Geometry: final body of the model. Coordinates: model frame, mm. A direction names the side the tool comes from. Round coordinates to 2 decimals unless told otherwise and drop trailing zeros. Loops run counter-clockwise (first coordinate to the right, second up) from the corner with the lowest first, then second, coordinate; pieces in that order, holes last. Notation, with made-up numbers: (33, 11.5) -> (66, 11.5) arc R26 ccw to (66, 50.5) -> close; hole circle Ø8 at (-8.75, -8.75). An arc over 180 degrees is marked (long way). Answer in a Markdown table with one row per item.
```python
from build123d import *

# Parameters (mm, degrees)
SKETCH_1_W             = 65
SKETCH_1_H             = 30
EXTRUDE_1_DEPTH        = 1.5
FILLET_1_R             = 3.5
SKETCH_2_R             = 1.375
CUT_EXTRUDE_1_DEPTH    = 1.5
SKETCH_3_R             = 3
CUT_EXTRUDE_2_DEPTH    = 0.1
CUT_EXTRUDE_3_REACH    = 37.826
SKETCH_5_R             = 0.25
PATTERN_LINEAR_1_COUNT = 20
PATTERN_LINEAR_1_PITCH = 2.54
SKETCH_6_W             = 11.2
SKETCH_6_H             = 7.1
SKETCH_6_W_2           = 7.9
SKETCH_6_H_2           = 5
EXTRUDE_3_DEPTH        = 3
SKETCH_7_W             = 12
SKETCH_7_H             = 12
EXTRUDE_4_DEPTH        = 1
SKETCH_8_W             = 11
SKETCH_8_H             = 11
EXTRUDE_5_DEPTH        = 1
SKETCH_9_W             = 1
SKETCH_9_H             = 7
CUT_EXTRUDE_4_DEPTH    = 1
SKETCH_4_W             = 51
SKETCH_4_H             = 5.5
SKETCH_4_W_2           = 50
SKETCH_4_H_2           = 4.5
CUT_EXTRUDE_5_DEPTH    = 0.1


with BuildPart() as part:
    # Sketch 1 → Extrude 1 (new body)
    with BuildSketch(Plane.XY):
        Rectangle(SKETCH_1_W, SKETCH_1_H)
    extrude(amount=EXTRUDE_1_DEPTH)

    # Fillet 1
    fillet_1_edges = [part.edges().sort_by_distance(p)[0] for p in [
        (-32.5, 15, 0.75),
        (32.5, 15, 0.75),
        (32.5, -15, 0.75),
        (-32.5, -15, 0.75),
    ]]
    fillet(fillet_1_edges, radius=FILLET_1_R)

    # Sketch 2 → Cut-Extrude 1 (cut)
    with BuildSketch(Plane.XY.offset(1.5)):
        with Locations((29, -11.5)):
            Circle(SKETCH_2_R)
        with Locations((29, 11.5)):
            Circle(SKETCH_2_R)
        with Locations((-29, -11.5)):
            Circle(SKETCH_2_R)
        with Locations((-29, 11.5)):
            Circle(SKETCH_2_R)
    extrude(amount=-CUT_EXTRUDE_1_DEPTH, mode=Mode.SUBTRACT)

    # Sketch 3 → Cut-Extrude 2 (cut)
    with BuildSketch(Plane.XY.offset(1.5)):
        with Locations((29, -11.5)):
            Circle(SKETCH_3_R)
        with Locations((29, 11.5)):
            Circle(SKETCH_3_R)
        with Locations((-29, -11.5)):
            Circle(SKETCH_3_R)
        with Locations((-29, 11.5)):
            Circle(SKETCH_3_R)
    extrude(amount=-CUT_EXTRUDE_2_DEPTH, mode=Mode.SUBTRACT)

    # Sketch 5 → Cut-Extrude 3 (cut, up to next)
    with BuildSketch(Plane.XY.offset(1.5), mode=Mode.PRIVATE) as cut_extrude_3_sk1:
        with Locations((24.13, -13.02)):
            Circle(SKETCH_5_R)
    cut_extrude_3_tool1 = extrude(cut_extrude_3_sk1.sketch, amount=-CUT_EXTRUDE_3_REACH, mode=Mode.PRIVATE) & part.part
    # Sketch 5 → Cut-Extrude 3 (cut, up to next)
    with BuildSketch(Plane.XY.offset(1.5), mode=Mode.PRIVATE) as cut_extrude_3_sk2:
        with Locations((24.13, -10.48)):
            Circle(SKETCH_5_R)
    cut_extrude_3_tool2 = extrude(cut_extrude_3_sk2.sketch, amount=-CUT_EXTRUDE_3_REACH, mode=Mode.PRIVATE) & part.part
    cut_extrude_3_1 = cut_extrude_3_tool1.solids().sort_by_distance((24.13, -13.02, 1.5))[0]
    add(cut_extrude_3_1, mode=Mode.SUBTRACT)
    cut_extrude_3_2 = cut_extrude_3_tool2.solids().sort_by_distance((24.13, -10.48, 1.5))[0]
    add(cut_extrude_3_2, mode=Mode.SUBTRACT)
    cut_extrude_3 = cut_extrude_3_1 + cut_extrude_3_2  # Cut-Extrude 3 as one shape, for the pattern or mirror that repeats it

    # Pattern Linear 1: Cut-Extrude 3 ×20
    with Locations(*[(-i * PATTERN_LINEAR_1_PITCH, 0, 0) for i in range(1, PATTERN_LINEAR_1_COUNT)]):
        add(cut_extrude_3, mode=Mode.SUBTRACT)

    # Sketch 6 → Extrude 3 (add)
    with BuildSketch(Plane.XY.offset(1.5)):
        with Locations((20.1, 11.95)):
            Rectangle(SKETCH_6_W, SKETCH_6_H)
        with Locations((-8.9, 13.5)):
            Rectangle(SKETCH_6_W_2, SKETCH_6_H_2)
        with Locations((-21.5, 13.5)):
            Rectangle(SKETCH_6_W_2, SKETCH_6_H_2)
    extrude(amount=EXTRUDE_3_DEPTH)

    # Sketch 7 → Extrude 4 (add)
    with BuildSketch(Plane.XY.offset(1.5)):
        with Locations((6.5, 2)):
            Rectangle(SKETCH_7_W, SKETCH_7_H)
    extrude(amount=EXTRUDE_4_DEPTH)

    # Sketch 8 → Extrude 5 (add)
    with BuildSketch(Plane.XY.offset(1.5)):
        with Locations((26, -1.9)):
            Rectangle(SKETCH_8_W, SKETCH_8_H)
    extrude(amount=EXTRUDE_5_DEPTH)

    # Sketch 9 → Cut-Extrude 4 (cut)
    with BuildSketch(Plane.XY.offset(2.5)):
        with Locations((31, -1.9)):
            Rectangle(SKETCH_9_W, SKETCH_9_H)
    extrude(amount=-CUT_EXTRUDE_4_DEPTH, mode=Mode.SUBTRACT)

    # Sketch 4 → Cut-Extrude 5 (cut)
    with BuildSketch(Plane.XY.offset(1.5)):
        with Locations((0, -11.75)):
            Rectangle(SKETCH_4_W, SKETCH_4_H)
        with Locations((0, -11.75)):
            Rectangle(SKETCH_4_W_2, SKETCH_4_H_2, mode=Mode.SUBTRACT)
    extrude(amount=-CUT_EXTRUDE_5_DEPTH, mode=Mode.SUBTRACT)


solid = part.part
```
Item 1: Ray query, L1, parallel to Y at x = -16.51, z = 0.95; L2, parallel to Z at x = 7, y = 3.5; L3, parallel to Z at x = -14, y = 14.5. Return the intervals inside material, ascending.
Ans:
| item | result |
|---|---|
| L1 | -15 to -13.27, -12.77 to -10.73, -10.23 to 15 |
| L2 | 0 to 2.5 |
| L3 | 0 to 1.5 |
Item 2: Section query B-B, the plane x = 10. Output: boundary loops of the cut face in (y, z).
Ans:
| item | result |
|---|---|
| outline | (-15, 0) -> (15, 0) -> (15, 1.5) -> (8, 1.5) -> (8, 2.5) -> (-4, 2.5) -> (-4, 1.5) -> (-9, 1.5) -> (-9, 1.4) -> (-9.5, 1.4) -> (-9.5, 1.5) -> (-14, 1.5) -> (-14, 1.4) -> (-14.5, 1.4) -> (-14.5, 1.5) -> (-15, 1.5) -> close |
Item 3: Section query A-A, the plane z = 3.4. Output: boundary loops of the cut face in (x, y), and give its area (3 significant figures).
Ans:
| item | result |
|---|---|
| outline | (-25.45, 11) -> (-17.55, 11) -> (-17.55, 16) -> (-25.45, 16) -> close; (-12.85, 11) -> (-4.95, 11) -> (-4.95, 16) -> (-12.85, 16) -> close; (14.5, 8.4) -> (25.7, 8.4) -> (25.7, 15.5) -> (14.5, 15.5) -> close |
| area | 159 mm2 |
Item 4: Section query D-D, the plane x = -7.5. Output: boundary loops of the cut face in (y, z).
Ans:
| item | result |
|---|---|
| outline | (-15, 0) -> (15, 0) -> (15, 1.5) -> (16, 1.5) -> (16, 4.5) -> (11, 4.5) -> (11, 1.5) -> (-9, 1.5) -> (-9, 1.4) -> (-9.5, 1.4) -> (-9.5, 1.5) -> (-14, 1.5) -> (-14, 1.4) -> (-14.5, 1.4) -> (-14.5, 1.5) -> (-15, 1.5) -> close |
Item 5: Mould query, pull axis X, two halves, no side actions, for faces 5 (the flat face through (-32.5, 0, 1)), 6 (the flat face through (-9, 14, 4.5)), 7 (the flat face through (14.5, 12, 3)). Classes: released by +X, released by -X, zero draft, split by the parting line, or undercut.
Ans:
| item | result |
|---|---|
| face 5 | released by -X |
| face 6 | zero draft |
| face 7 | undercut |
Item 6: Set-up query: faces 1 (the flat face through (20, 15.5, 3)), 2 (the flat face through (20, 8.4, 3)), 3 (the flat face through (-28, 10, 1.4)), 4 (the flat face through (0, 15, 1)). Return all of +Z, -Z, +X, -X, +Y, -Y with unobstructed straight access to the full face (end or side cutting, diameter ignored); none if empty.
Ans:
| item | result |
|---|---|
| face 1 | +Z, -Z, +X, +Y |
| face 2 | +Z, +X, -X |
| face 3 | +Z |
| face 4 | -Z, +X, -X, +Y |
Item 7: First-contact query: P1, Ø2.5, axis at y = 14.5, z = 2.5, coming from the -X side; P2, Ø0.9, axis at y = 14.5, z = 3.5, coming from the -X side; P3, Ø1, axis at x = 21, y = 6, coming from the +Z side. Flat tips, straight axial feed; report the tip coordinate or a pass-through.
Ans:
| item | result |
|---|---|
| P1 | x = -31.68 |
| P2 | x = -25.45 |
| P3 | z = 1.5 |
Item 8: Section query C-C, the plane y = 7. Output: boundary loops of the cut face in (x, z).
Ans:
| item | result |
|---|---|
| outline | (-32.5, 0) -> (32.5, 0) -> (32.5, 1.5) -> (12.5, 1.5) -> (12.5, 2.5) -> (0.5, 2.5) -> (0.5, 1.5) -> (-32.5, 1.5) -> close |
